Can you work these out from the model? Positions are in its coordinate system, mm. Face numbers are marked on the shaded views. A direction names the side the tool comes from. Give positions to 0.01 mm unless a question says otherwise; leave off trailing zeros. Order: outer loops, then holes, each group sorted by start corner. A loop starts at its lowest first (then second) coordinate and runs counter-clockwise, first axis right, second up. Notation, with made-up numbers: (1.5, -8) - (55.5, -8) arc R18 cw to (55.5, 10) - close; hole circle Ø10 at (63.5, 1). An arc over 180 degrees is marked (long way). One line per question, with ' | ' between items.
```python
from build123d import *

# Parameters (mm, degrees)
BOSS_EXTRUDE1_DEPTH      = 54
BOSS_EXTRUDE2_DEPTH      = 54
CUT_EXTRUDE4_DEPTH       = 79.958686857
CUT_EXTRUDE8_DEPTH       = 120
CUT_EXTRUDE8_DEPTH_BACK  = 57
SKETCH4_R                = 4
CUT_EXTRUDE10_DEPTH      = 155
CUT_EXTRUDE10_DEPTH_BACK = 93
SKETCH5_R                = 4
CUT_EXTRUDE11_DEPTH      = 155
SKETCH7_W                = 62.578276035
SKETCH7_H                = 34.481752036
SKETCH7_W_2              = 74.024148658
SKETCH7_H_2              = 32.895468992
CUT_EXTRUDE12_DEPTH      = 2


with BuildPart() as part:
    # Sketch1 → Boss-Extrude1 (new body)
    with BuildSketch(Plane.XY):
        Polygon((-95, 0), (87.264140028, 0), (84.264140028, 11), (-92, 11), align=None)
    extrude(amount=BOSS_EXTRUDE1_DEPTH)

    # Sketch2 → Boss-Extrude2 (add)
    with BuildSketch(Plane(origin=(0, 11, 0), x_dir=(1, 0, 0), z_dir=(0, 1, 0))):
        with BuildLine():
            Line((-37.334331048, -54), (29.598471075, -54))
            ThreePointArc((29.598471075, -54), (36.678680511, -41.3168564), (39.132070014, -27))
            ThreePointArc((39.132070014, -27), (36.678680511, -12.6831436), (29.598471075, 0))
            Line((29.598471075, 0), (-37.334331048, 0))
            ThreePointArc((-37.334331048, 0), (-46.867929986, -27), (-37.334331048, -54))
        make_face()
    extrude(amount=BOSS_EXTRUDE2_DEPTH)

    # Sketch3 → Cut-Extrude4 (cut, symmetric)
    with BuildSketch(Plane.XY):
        with BuildLine():
            Line((15.132070014, 52), (18.132070014, 52))
            Line((18.132070014, 52), (18.132070014, 65))
            Line((18.132070014, 65), (-25.867929986, 65))
            Line((-25.867929986, 65), (-25.867929986, 52))
            Line((-25.867929986, 52), (-22.867929986, 52))
            ThreePointArc((-22.867929986, 52), (-3.867929986, 33), (15.132070014, 52))
        make_face()
    extrude(amount=CUT_EXTRUDE4_DEPTH, both=True, mode=Mode.SUBTRACT)

    # Sketch4 → Cut-Extrude8 (cut, two sides: drawn at the far end of the back side and taken through both)
    with BuildSketch(Plane(origin=(0, 0, 0), x_dir=(1, 0, 0), z_dir=(0, 1, 0)).offset(-CUT_EXTRUDE8_DEPTH_BACK)):
        with Locations(Location((-34.646506606, -27, 0), (0, 0, 270))):
            Circle(SKETCH4_R)
    extrude(amount=CUT_EXTRUDE8_DEPTH + CUT_EXTRUDE8_DEPTH_BACK, mode=Mode.SUBTRACT)

    # Sketch5 → Cut-Extrude10 (cut, two sides: drawn at the far end of the back side and taken through both)
    with BuildSketch(Plane(origin=(0, 0, 0), x_dir=(1, 0, 0), z_dir=(0, 1, 0)).offset(-CUT_EXTRUDE10_DEPTH_BACK)):
        with Locations(Location((26.963039677, -27, 0), (0, 0, 270))):
            Circle(SKETCH5_R)
    extrude(amount=CUT_EXTRUDE10_DEPTH + CUT_EXTRUDE10_DEPTH_BACK, mode=Mode.SUBTRACT)

    # Sketch6 → Cut-Extrude11 (cut)
    with BuildSketch(Plane(origin=(0, 11, 0), x_dir=(1, 0, 0), z_dir=(0, 1, 0))):
        with BuildLine():
            Line((75, -32), (59, -32))
            ThreePointArc((59, -32), (54, -27), (59, -22))
            Line((59, -22), (75, -22))
            ThreePointArc((75, -22), (80, -27), (75, -32))
        make_face()
        with BuildLine():
            Line((-59, -32), (-75, -32))
            ThreePointArc((-75, -32), (-80, -27), (-75, -22))
            Line((-75, -22), (-59, -22))
            ThreePointArc((-59, -22), (-54, -27), (-59, -32))
        make_face()
    extrude(amount=-CUT_EXTRUDE11_DEPTH, mode=Mode.SUBTRACT)

    # Sketch7 → Cut-Extrude12 (cut)
    with BuildSketch(Plane.XZ):
        with Locations((-52.436526345, 25.989630072)):
            Rectangle(SKETCH7_W, SKETCH7_H)
        with Locations((46.961370867, 26.782771594)):
            Rectangle(SKETCH7_W_2, SKETCH7_H_2)
    extrude(amount=-CUT_EXTRUDE12_DEPTH, mode=Mode.SUBTRACT)


solid = part.part
```
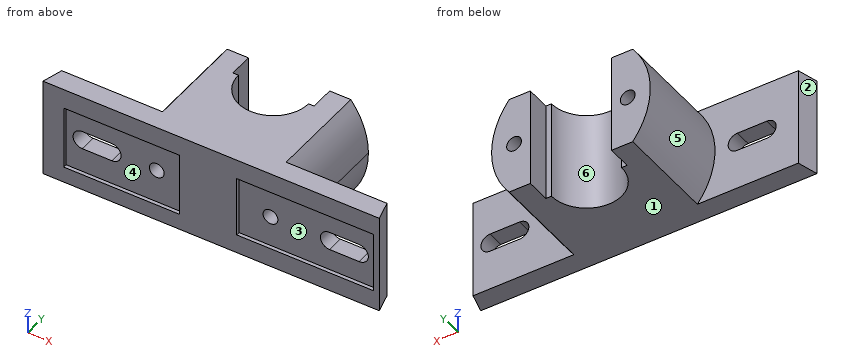
(1) Imagine slicing it at A-A (y = 15). List the corners of the cut face in (x, z) for me, and give its area (3 significant figures).
Answer below:
outline: (-37.33, 0) - (29.6, 0) arc R43 ccw to (29.6, 54) - (-37.33, 54) arc R43 ccw to start; hole circle Ø8 at (-34.65, 27); hole circle Ø8 at (26.96, 27) | area: 4,220 mm^2
(2) Imagine slicing it at B-B (z = 46). List the corners of the cut face in (x, y) for me, and give its area (3 significant figures).
Answer below:
outline: (-95, 0) - (87.26, 0) - (84.26, 11) - (34.71, 11) - (34.71, 65) - (18.13, 65) - (18.13, 52) - (15.13, 52) arc R19 cw to (-22.87, 52) - (-25.87, 52) - (-25.87, 65) - (-42.44, 65) - (-42.44, 11) - (-92, 11) - close | area: 5,000 mm^2
(3) If I drill on line 1 (X direction, y = 42, z = 28.5); line 2 (Y direction, x = -79, z = 41); line 3 (Y direction, x = 69, z = 48), over which ranges is the centre line in solid material (lowest first)?
Answer below:
line 1: -46.84 to -38.35, -30.94 to -20.02, 12.29 to 23.25, 30.67 to 39.11 | line 2: 2 to 11 | line 3: 0 to 11
(4) Imagine slicing it at D-D (z = 7). List the corners of the cut face in (x, y) for me.
Answer below:
outline: (-95, 0) - (87.26, 0) - (84.26, 11) - (34.2, 11) - (34.2, 65) - (18.13, 65) - (18.13, 52) - (15.13, 52) arc R19 cw to (-22.87, 52) - (-25.87, 52) - (-25.87, 65) - (-41.93, 65) - (-41.93, 11) - (-92, 11) - close
(5) Imagine slicing it at C-C (y = 6). List the corners of the cut face in (x, z) for me, and give its area (3 significant figures).
Answer below:
outline: (-93.36, 0) - (85.63, 0) - (85.63, 54) - (-93.36, 54) - close; hole (-75, 22) - (-59, 22) arc R5 ccw to (-59, 32) - (-75, 32) arc R5 ccw to start; hole circle Ø8 at (-34.65, 27); hole circle Ø8 at (26.96, 27); hole (59, 22) - (75, 22) arc R5 ccw to (75, 32) - (59, 32) arc R5 ccw to start | area: 9,090 mm^2
(6) Will these pins go through, and if not, where does the flat tip stop? pin 1 (16.5 mm diameter, centred on x = 48, z = 23, fed in from -Y); pin 2 (10 mm diameter, centred on y = 34, z = 24.5, fed in from -X); pin 3 (1 mm diameter, centred on y = 1, z = 21.5, fed in from +X); pin 4 (6.5 mm diameter, centred on x = -34.65, z = 27, fed in from -Y).
Answer below:
pin 1: y = 2 | pin 2: x = -46.87 | pin 3: x = 87.13 | pin 4: through
(7) On a 3-axis mill with a long thin cutter (end or side, diameter ignored), from which of +Z, -Z, +X, -X, +Y, -Y can I reach the whole of each face in a straight line? I mean the marked faces 5 and 6. Say none if no direction works.
Answer below:
face 5: -X, +Y | face 6: +Z, -Z, +Y
(8) If we mould it in two halves opening along Z, with no side actions, what happens to the marked faces 1, 2, 3 and 4? For each: released by +Z, released by -Z, zero draft, split by the parting line, or undercut.
Answer below:
face 1: released by -Z | face 2: zero draft | face 3: undercut | face 4: undercut
